```python
from build123d import *

# Parameters (mm, degrees)
SZKIC1_W                    = 104.872117299
SZKIC1_H                    = 113.043153049
SZKIC1_R                    = 8.139229877
DODANIE_WYCI_GNI_CIE1_DEPTH = 20
SZKIC2_R                    = 14.315912416
WYTNIJ_WYCI_GNI_CIE1_DEPTH  = 2
WYTNIJ_WYCI_GNI_CIE2_DEPTH  = 140
SZKIC9_R                    = 6.34096602
DODANIE_WYCI_GNI_CIE2_DEPTH = 60
SZKIC12_W                   = 26.801545634
SZKIC12_H                   = 113.043153049
WYTNIJ_WYCI_GNI_CIE8_DEPTH  = 99
SZKIC13_W                   = 18.676589494
SZKIC13_H                   = 43.251049354
WYTNIJ_WYCI_GNI_CIE9_DEPTH  = 85


with BuildPart() as part:
    # Szkic1 → Dodanie-wyciągnięcie1 (new body)
    with BuildSketch(Plane.XY):
        with Locations((-52.43605865, 6.459608746)):
            Rectangle(SZKIC1_W, SZKIC1_H)
        with Locations((-84.996398081, 6.459608746)):
            Circle(SZKIC1_R, mode=Mode.SUBTRACT)
    dodanie_wyci_gni_cie1 = extrude(amount=DODANIE_WYCI_GNI_CIE1_DEPTH)

    # Szkic2 → Wytnij-wyciągnięcie1 (cut)
    with BuildSketch(Plane.XY.offset(20)):
        with Locations((-84.996398081, 6.459608746)):
            Circle(SZKIC2_R)
    wytnij_wyci_gni_cie1 = extrude(amount=-WYTNIJ_WYCI_GNI_CIE1_DEPTH, mode=Mode.SUBTRACT)

    # Lustro2: Dodanie-wyciągnięcie1, Wytnij-wyciągnięcie1 across plane
    add(dodanie_wyci_gni_cie1.mirror(Plane(origin=(0, 62.98118527, 20), x_dir=(0, 0, 1), z_dir=(-1, 0, 0))))
    add(wytnij_wyci_gni_cie1.mirror(Plane(origin=(0, 62.98118527, 20), x_dir=(0, 0, 1), z_dir=(-1, 0, 0))), mode=Mode.SUBTRACT)

    # Szkic6 → Wytnij-wyciągnięcie2 (cut)
    with BuildSketch(Plane(origin=(0, 62.98118527, 0), x_dir=(1, 0, 0), z_dir=(0, 1, 0))):
        with BuildLine():
            Line((-23.533046442, 0), (23.533046442, 0))
            ThreePointArc((23.533046442, 0), (21.432956346, -4.78054627), (16.491575681, -6.467780152))
            Line((16.491575681, -6.467780152), (-16.491575681, -6.467780152))
            ThreePointArc((-16.491575681, -6.467780152), (-21.432956346, -4.78054627), (-23.533046442, 0))
        make_face()
    extrude(amount=-WYTNIJ_WYCI_GNI_CIE2_DEPTH, mode=Mode.SUBTRACT)

    # Szkic9 → Dodanie-wyciągnięcie2 (add)
    with BuildSketch(Plane(origin=(0, 0, 0), x_dir=(0, 0, -1), z_dir=(1, 0, 0))):
        with BuildLine():
            Line((-20, 62.98118527), (-72.068850924, 62.98118527))
            ThreePointArc((-72.068850924, 62.98118527), (-87.508244639, 53.371610982), (-85.703573327, 35.27570101))
            Line((-85.703573327, 35.27570101), (-20, -50.061967779))
            Line((-20, -50.061967779), (-20, 62.98118527))
        make_face()
        with Locations((-72.068850924, 45.773409652)):
            Circle(SZKIC9_R, mode=Mode.SUBTRACT)
    dodanie_wyci_gni_cie2 = extrude(amount=DODANIE_WYCI_GNI_CIE2_DEPTH)

    # Lustro3: Dodanie-wyciągnięcie2 across plane
    add(dodanie_wyci_gni_cie2.mirror(Plane(origin=(0, 45.773409652, 72.068850924), x_dir=(0, 0, 1), z_dir=(1, 0, 0))))

    # Szkic12 → Wytnij-wyciągnięcie8 (cut)
    with BuildSketch(Plane.XY.offset(35)):
        with Locations((0, 6.459608746)):
            Rectangle(SZKIC12_W, SZKIC12_H)
    extrude(amount=WYTNIJ_WYCI_GNI_CIE8_DEPTH, mode=Mode.SUBTRACT)

    # Szkic13 → Wytnij-wyciągnięcie9 (cut)
    with BuildSketch(Plane.XY.offset(35)):
        with Locations((0, -46.989841451)):
            Rectangle(SZKIC13_W, SZKIC13_H)
    extrude(amount=-WYTNIJ_WYCI_GNI_CIE9_DEPTH, mode=Mode.SUBTRACT)


solid = part.part
```
Read the model definition and answer for the solid it produces. Units are mm, in the model's axes. A direction names the side the tool comes from. Give positions to 0.01 mm unless a question says otherwise; leave off trailing zeros. Order: outer loops, then holes, each group sorted by start corner. A loop starts at its lowest first (then second) coordinate and runs counter-clockwise, first axis right, second up. Notation, with made-up numbers: (62.5, -3) -> (74.5, -3) arc R32 cw to (74.5, 35) -> close; hole circle Ø10 at (-3, 17.5). An arc over 180 degrees is marked (long way). Write item = value, one per line.
1. For faces 1 (the face through (-9.338, -35, 18)), 2 (the face through (13.401, 26, 56)), 3 (the face through (-71.77, 0.98, 19.01)), 4 (the face through (0, 7, 6.468)), determine the directions among +Z, -Z, +X, -X, +Y, -Y from which every point of the face is accessible in a straight line to the end or side of a thin tool.
Numbers:
face_1 = +Z, -Z, -Y
face_2 = +Z, +Y, -Y
face_3 = +Z
face_4 = -Z, +Y, -Y
2. Straight lines are drawn through the part: line 1 along X through (y, z) = (57, 60); line 2 along Z through (x, y) = (-8, -14); line 3 along Z through (x, y) = (-80, 57.5). For each, find the intervals that lie inside material, in ascending order.
Numbers:
line_1 = -60 to -13.4, 13.4 to 60
line_2 = 6.47 to 35
line_3 = 0 to 20
3. A cutting plane is placed at C-C, the plane x = -21. Write down the section's boundary in (y, z).
Numbers:
outline = (-50.06, 5.14) -> (62.98, 5.14) -> (62.98, 72.07) arc R17.21 ccw to (35.28, 85.7) -> (-50.06, 20) -> close; hole circle Ø12.68 at (45.77, 72.07)
4. A cutting plane is placed at D-D, the plane y = -17. Write down the section's boundary in (x, z), and give its area (3 significant figures).
Numbers:
outline = (-104.87, 0) -> (-23.53, 0) arc R6.49 cw to (-16.49, 6.47) -> (16.49, 6.47) arc R6.49 cw to (23.53, 0) -> (104.87, 0) -> (104.87, 20) -> (60, 20) -> (60, 45.46) -> (13.4, 45.46) -> (13.4, 35) -> (-13.4, 35) -> (-13.4, 45.46) -> (-60, 45.46) -> (-60, 20) -> (-104.87, 20) -> close
area = 6,680 mm²
5. A cutting plane is placed at B-B, the plane z = 10.5. Write down the section's boundary in (x, y).
Numbers:
outline = (-104.87, -50.06) -> (-9.34, -50.06) -> (-9.34, -25.36) -> (9.34, -25.36) -> (9.34, -50.06) -> (104.87, -50.06) -> (104.87, 62.98) -> (-104.87, 62.98) -> close; hole circle Ø16.28 at (-85, 6.46); hole circle Ø16.28 at (85, 6.46)
6. A cutting plane is placed at A-A, the plane z = 49. Write down the section's boundary in (x, y), and give its area (3 significant figures).
Numbers:
outline = (-60, -12.4) -> (-13.4, -12.4) -> (-13.4, 62.98) -> (-60, 62.98) -> close; (13.4, -12.4) -> (60, -12.4) -> (60, 62.98) -> (13.4, 62.98) -> close
area = 7,030 mm²
7. Given pin 1 (22.5 mm diameter, centred on x = 89.5, y = -2, fed in from +Z); pin 2 (5 mm diameter, centred on x = -9, z = 26.5, fed in from -Y); pin 3 (6 mm diameter, centred on y = 12, z = 39.5, fed in from +X), each flat-ended and moving along its own axis, determine where each tip first touches the part or whether it passes through.
Numbers:
pin_1 = 20
pin_2 = -44.84
pin_3 = 60
8. The mould has two halves that part along Y. Classify faces 5 (the face through (0, -25.364, 21)), 6 (the face through (93.128, 6.817, 8.874)), 7 (the face through (-77, 20, 20)), 8 (the face through (71.77, 0.98, 19.01)): +Y half, -Y half, draft (parallel to the pull), parting line (faces both ways), or undercut.
Numbers:
face_5 = -Y half
face_6 = undercut
face_7 = draft
face_8 = undercut
